```python
from build123d import *

# Parameters (mm, degrees)
SKETCH_1_W                  = 32
SKETCH_1_H                  = 32
EXTRUDE_1_DEPTH             = 3
HOLE_WIZARD_3_4_3_4_1_D     = 3.4
HOLE_WIZARD_3_4_3_4_1_DEPTH = 6
HOLE_WIZARD_3_4_3_4_1_TIP   = 1.021463052
PATTERN_CIRCULAR_1_COUNT    = 4
HOLE_WIZARD_M4_1_D          = 3.3
CHAMFER_1_SIZE              = 1


with BuildPart() as part:
    # 草图1 → 凸台-拉伸1 (new body)
    with BuildSketch(Plane.XY):
        with Locations((0, -3)):
            Rectangle(SKETCH_1_W, SKETCH_1_H)
    extrude(amount=EXTRUDE_1_DEPTH)

    # Ø3.4 (3.4) 直径孔1
    with Locations(Plane.XY.offset(3)):
        with Locations((0, 0)):
            Hole(HOLE_WIZARD_3_4_3_4_1_D / 2, depth=HOLE_WIZARD_3_4_3_4_1_DEPTH)
            with Locations((0, 0, -(HOLE_WIZARD_3_4_3_4_1_DEPTH + HOLE_WIZARD_3_4_3_4_1_TIP / 2))):  # 118° drill point
                Cone(0, HOLE_WIZARD_3_4_3_4_1_D / 2, HOLE_WIZARD_3_4_3_4_1_TIP, mode=Mode.SUBTRACT)

    # 草图4 → M3 螺纹孔1 (revolve, cut)
    with BuildSketch(Plane(origin=(-4.949747468, -4.949747468, 3), x_dir=(0, -1, 0), z_dir=(1, 0, 0))):
        Polygon((0, 0), (0, 9.251075774), (1.25, 8.5), (1.25, 0), align=None)
    hole_wizard_m3_1 = revolve(axis=Axis((-4.949747468, -4.949747468, 9.35), (0, 0, -1)), mode=Mode.SUBTRACT)

    # 阵列(圆周)1: M3 螺纹孔1 ×4 about axis
    pattern_circular_1_axis = Axis((0, 0, 0), (0, 0, 1))
    for i in range(1, PATTERN_CIRCULAR_1_COUNT):
        add(hole_wizard_m3_1.rotate(pattern_circular_1_axis, i * 360 / PATTERN_CIRCULAR_1_COUNT), mode=Mode.SUBTRACT)

    # M4 螺纹孔1 (through all)
    with Locations(Plane.XY.offset(3)):
        with Locations((-11, 8), (11, 8), (-11, -15.5), (11, -15.5)):
            Hole(HOLE_WIZARD_M4_1_D / 2)

    # 倒角1
    chamfer_1_edges = [part.edges().sort_by_distance(p)[0] for p in [
        (-16, 13, 1.5),
        (16, 13, 1.5),
        (16, -19, 1.5),
        (-16, -19, 1.5),
    ]]
    chamfer(chamfer_1_edges, length=CHAMFER_1_SIZE)


solid = part.part
```
Check sheet for the modelled part. Datum: model origin and axes. Units: mm. Round coordinates to 2 decimals unless told otherwise and drop trailing zeros. Order: outer loops, then holes, each group sorted by start corner. A loop starts at its lowest first (then second) coordinate and runs counter-clockwise, first axis right, second up. Notation, with made-up numbers: (-19.75, -14) - (-15.75, -14) arc R10 cw to (-15.75, -1) - close; hole circle Ø11 at (28.25, -4.75). An arc over 180 degrees is marked (long way). Write item = value, one per line.
Q1. Section check B-B (x = 0). Record the boundary of the cut face in (y, z).
Computed:
outline = (-19, 0) - (-1.7, 0) - (-1.7, 3) - (-19, 3) - close; (1.7, 0) - (13, 0) - (13, 3) - (1.7, 3) - close
Q2. Section check D-D (y = 0). Record the boundary of the cut face in (x, z), and give its area (3 significant figures).
Computed:
outline = (-16, 0) - (-1.7, 0) - (-1.7, 3) - (-16, 3) - close; (1.7, 0) - (16, 0) - (16, 3) - (1.7, 3) - close
area = 85.8 mm^2
Q3. Thickness scan on line 1 along Y through (x, z) = (-11, 1.45); line 2 along Y through (x, z) = (-5, 1.15); line 3 along X through (y, z) = (-16, 0.35). Record the ranges inside material, lowest first.
Computed:
line_1 = -19 to -17.15, -13.85 to 6.35, 9.65 to 13
line_2 = -19 to -6.2, -3.7 to 3.7, 6.2 to 13
line_3 = -16 to -12.57, -9.43 to 9.43, 12.57 to 16
Q4. Draft check along Y on faces 1 (the face through (16, -3, 1)), 2 (the face through (-3.73, -4.68, 1.52)), 3 (the face through (0, -19, 1)), 4 (the face through (0, 13, 1)). Enter one of: pulls with the +Y half, pulls with the -Y half, needs draft (parallel to the pull), parting line crosses it, or undercut.
Computed:
face_1 = needs draft
face_2 = undercut
face_3 = pulls with the -Y half
face_4 = pulls with the +Y half
Q5. Section check C-C (x = -11). Record the boundary of the cut face in (y, z), and give its area (3 significant figures).
Computed:
outline = (-19, 0) - (-17.15, 0) - (-17.15, 3) - (-19, 3) - close; (-13.85, 0) - (6.35, 0) - (6.35, 3) - (-13.85, 3) - close; (9.65, 0) - (13, 0) - (13, 3) - (9.65, 3) - close
area = 76.2 mm^2
Q6. Go/stop test with a flat-tipped pin: pin 1 (2 mm diameter, centred on x = -4.95, y = 4.95, fed in from +Z). Record where the tip stops, or that it passes through.
Computed:
pin_1 = through
Q7. Section check A-A (y = 8). Record the boundary of the cut face in (x, z).
Computed:
outline = (-16, 0) - (-12.65, 0) - (-12.65, 3) - (-16, 3) - close; (-9.35, 0) - (9.35, 0) - (9.35, 3) - (-9.35, 3) - close; (12.65, 0) - (16, 0) - (16, 3) - (12.65, 3) - close
